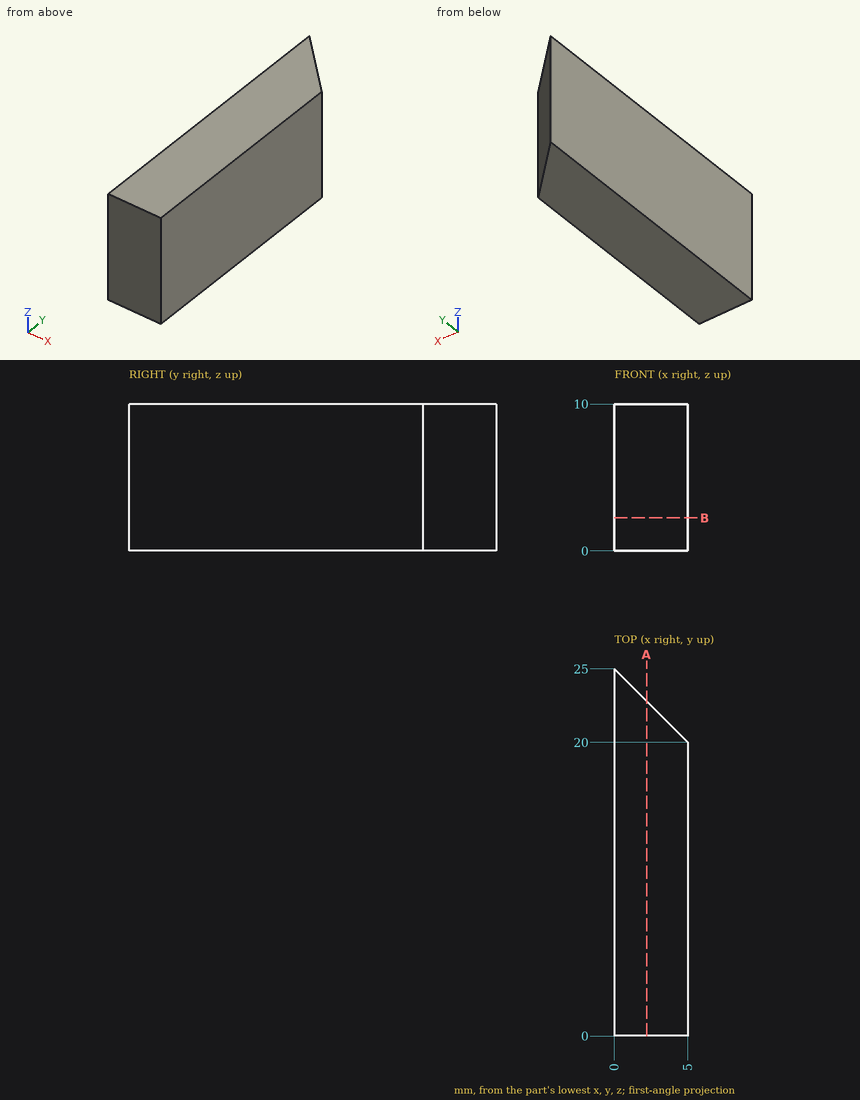
Could you check a few things on this drawing? It's one solid part, dimensions in mm from its lowest x, y, z. Coordinates: 2 decimals unless noted, no trailing zeros. Order: outer loops, then holes, each group sorted by start corner. A loop starts at its lowest first (then second) coordinate and runs counter-clockwise, first axis right, second up. Notation, with made-up numbers: (67.5, 7.25) - (85.5, 7.25) arc R27 cw to (85.5, 46.25) - close; hole circle Ø2 at (61.5, -24). An arc over 180 degrees is marked (long way). Answer as a JSON object with one key per item and string values. Group by question number.
Q1. Imagine slicing it at B-B (z = 2.25). Please give me the cut outline in (x, y), and give its area (4 significant figures).
Q2. Imagine slicing it at A-A (x = 2.2). Please give me the cut outline in (y, z), and give its area (3 significant figures).
Q3. I need wall thicknesses on line 1 (Y direction, x = 3.2, z = 8.5); line 2 (Y direction, x = 0.7, z = 3); line 3 (X direction, y = 21, z = 4). Which ranges of each line are inside material? Lowest first, please. Write a range as from..to.
Determined:
{
 "1": {"outline": "(0, 0) - (5, 0) - (5, 20) - (0, 25) - close", "area": "112.5 mm2"},
 "2": {"outline": "(0, 0) - (22.8, 0) - (22.8, 10) - (0, 10) - close", "area": "228 mm2"},
 "3": {"line 1": "y = 0..21.8", "line 2": "y = 0..24.3", "line 3": "x = 0..4"}
}
